from build123d import *

# Parameters (mm, degrees)
IZIM1_W                     = 50
IZIM1_H                     = 80
Y_KSEKLIK_EKSTR_ZYON2_DEPTH = 60
IZIM2_W                     = 15
IZIM2_H                     = 12
Y_KSEKLIK_EKSTR_ZYON3_DEPTH = 12
AYNALAMA2_COPY_1_SKETCH_W   = 15
AYNALAMA2_COPY_1_SKETCH_H   = 12
AYNALAMA2_COPY_1_DEPTH      = 12
KES_EKSTR_ZYON1_DEPTH       = 50


with BuildPart() as part:
    # Çizim1 → Yükseklik-Ekstrüzyon2 (new body)
    with BuildSketch(Plane(origin=(0, 0, 0), x_dir=(1, 0, 0), z_dir=(0, 1, 0))):
        Rectangle(IZIM1_W, IZIM1_H)
    extrude(amount=Y_KSEKLIK_EKSTR_ZYON2_DEPTH)

    # Çizim2 → Yükseklik-Ekstrüzyon3 (add)
    with BuildSketch(Plane.XY.offset(40)):
        with Locations((-17.5, 6)):
            Rectangle(IZIM2_W, IZIM2_H)
    y_kseklik_ekstr_zyon3 = extrude(amount=Y_KSEKLIK_EKSTR_ZYON3_DEPTH)

    # Aynalama1: Yükseklik-Ekstrüzyon3 across plane
    add(y_kseklik_ekstr_zyon3.mirror(Plane(origin=(0, 0, 0), x_dir=(0, 0, 1), z_dir=(1, 0, 0))))

    # Aynalama2: Yükseklik-Ekstrüzyon3 across plane
    add(y_kseklik_ekstr_zyon3.mirror(Plane.XY))

    # Aynalama2 copy 1 sketch → Aynalama2 copy 1 (add)
    with BuildSketch(Plane(origin=(0, 0, -40), x_dir=(-1, 0, 0), z_dir=(0, 0, -1))):
        with Locations((-17.5, 6)):
            Rectangle(AYNALAMA2_COPY_1_SKETCH_W, AYNALAMA2_COPY_1_SKETCH_H)
    extrude(amount=AYNALAMA2_COPY_1_DEPTH)

    # Çizim3 → Kes-Ekstrüzyon1 (cut)
    with BuildSketch(Plane.XY.offset(25)):
        Polygon((-10, 60), (25, 25), (25, 60), align=None)
    extrude(amount=-KES_EKSTR_ZYON1_DEPTH, mode=Mode.SUBTRACT)


solid = part.part
Input: part model. Units: mm. Frame: model coordinates. A direction names the side the tool comes from. Round coordinates to 2 decimals unless told otherwise and drop trailing zeros. Write each loop counter-clockwise with the first axis right and the second up, starting at its lowest first coordinate (ties: lowest second). Pieces come first, ordered by that corner, then holes.
1) Cut plane A-A (y = 50.5). Return the cut outline in (x, z), then the cut area to 4 significant figures.
2) Contact query for flat-ended pins moving along their axis: P1, Ø17.5, axis at x = 13.5, y = 35.5, coming from the -Z side; P2, Ø1, axis at y = 43.5, z = -13.5, coming from the +X side; P3, Ø6, axis at x = 17.5, z = 48, coming from the +Y side. Output: stop coordinate, or through.
3) Cut plane C-C (z = 1.5). Return the cut outline in (x, y).
4) Cut plane D-D (y = 7). Return the cut outline in (x, z), then the cut area to 3 significant figures.
5) Cut plane B-B (x = -2). Return the cut outline in (y, z).
6) Ray query, L1, parallel to Z at x = 16, y = 55.5; L2, parallel to Z at x = -11.5, y = 41; L3, parallel to Y at x = -12, z = 41.5. Return the intervals inside material, ascending.
7) Reachability of faces 1 (the flat face through (10, 6, 46)), 2 (the flat face through (18, 12, 46)), 3 (the flat face through (18, 12, -46)), 4 (the flat face through (10, 6, -46)) from +Z, -Z, +X, -X, +Y, -Y: full face, straight path, thin tool, end or side. Return the list, or none.
8) Draft query along Z for faces 5 (the flat face through (7, 43, 0)), 6 (the flat face through (-18, 6, 52)), 7 (the flat face through (-18, 12, 46)), 8 (the flat face through (15, 51, 25)). Return one class per face: pulls with the +Z half, pulls with the -Z half, needs draft (parallel to the pull), parting line crosses it, or undercut.
Geometry says:
1. outline: (-25, -40) - (25, -40) - (25, -25) - (-0.5, -25) - (-0.5, 25) - (25, 25) - (25, 40) - (-25, 40) - close
1. area: 2,725 mm2
2. P1: stops at z = -40
2. P2: stops at x = 7
2. P3: stops at y = 12
3. outline: (-25, 0) - (25, 0) - (25, 25) - (-10, 60) - (-25, 60) - close
4. outline: (-25, -52) - (-10, -52) - (-10, -40) - (10, -40) - (10, -52) - (25, -52) - (25, 52) - (10, 52) - (10, 40) - (-10, 40) - (-10, 52) - (-25, 52) - close
4. area: 4,720 mm2
5. outline: (0, -40) - (60, -40) - (60, -25) - (52, -25) - (52, 25) - (60, 25) - (60, 40) - (0, 40) - close
6. L1: z = -40 to -25, 25 to 40
6. L2: z = -40 to 40
6. L3: y = 0 to 12
7. face 1: +Z, +Y, -Y
7. face 2: +Z, +X, -X, +Y
7. face 3: -Z, +X, -X, +Y
7. face 4: -Z, +Y, -Y
8. face 5: undercut
8. face 6: pulls with the +Z half
8. face 7: needs draft
8. face 8: undercut
